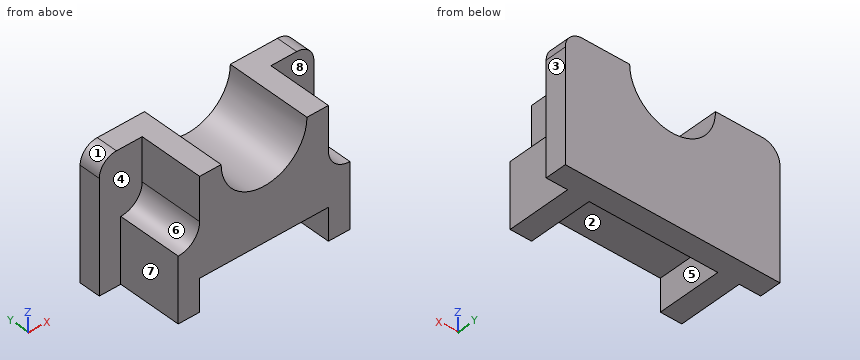
from build123d import *

# Parameters (mm, degrees)
F1_DEPTH = 6.35
F2_R     = 5.08
F4_DEPTH = 19.05
F5_DEPTH = 25.4
F6_DEPTH = 25.4
F7_DEPTH = 72.5614
F8_DEPTH = 61.46767


with BuildPart() as f1:
    # F0 (on Front) → F1 (new body)
    with BuildSketch(Plane.XZ):
        with BuildLine():
            Line((-25.4, 33.425663), (-44.45, 33.425663))
            Line((-44.45, 33.425663), (-44.45, -4.674337))
            Line((-44.45, -4.674337), (19.05, -4.674337))
            Line((19.05, -4.674337), (19.05, 33.425663))
            Line((19.05, 33.425663), (0, 33.425663))
            ThreePointArc((0, 33.425663), (-12.7, 20.725663), (-25.4, 33.425663))
        make_face()
        with BuildLine():
            Line((0, 33.425663), (-25.4, 33.425663))
            ThreePointArc((-25.4, 33.425663), (-12.7, 20.725663), (0, 33.425663))
        make_face()
    extrude(amount=F1_DEPTH)

    # F2
    f2_edges = [f1.edges().sort_by_distance(p)[0] for p in [
        (-44.45, -3.175, 33.425663),
        (19.05, -3.175, 33.425663),
    ]]
    fillet(f2_edges, radius=F2_R)

    # F3 (on face) → F4 (join)
    with BuildSketch(Plane.XZ.offset(6.35)):
        with BuildLine():
            Line((-38.1, 14.375663), (-38.1, -4.674337))
            Line((-38.1, -4.674337), (-31.75, -4.674337))
            Line((-31.75, -4.674337), (-31.75, 4.850663))
            Line((-31.75, 4.850663), (6.35, 4.850663))
            Line((6.35, 4.850663), (6.35, -4.674337))
            Line((6.35, -4.674337), (12.7, -4.674337))
            Line((12.7, -4.674337), (12.7, 14.375663))
            ThreePointArc((12.7, 14.375663), (8.209872, 16.235535), (6.35, 20.725663))
            Line((6.35, 20.725663), (6.35, 33.425663))
            Line((6.35, 33.425663), (-31.75, 33.425663))
            Line((-31.75, 33.425663), (-31.75, 20.725663))
            ThreePointArc((-31.75, 20.725663), (-33.609872, 16.235535), (-38.1, 14.375663))
        make_face()
        with BuildLine():
            Line((-38.1, 33.425663), (-38.1, 14.375663))
            ThreePointArc((-38.1, 14.375663), (-33.609872, 16.235535), (-31.75, 20.725663))
            Line((-31.75, 20.725663), (-31.75, 33.425663))
            Line((-31.75, 33.425663), (-38.1, 33.425663))
        make_face()
        with BuildLine():
            Line((12.7, 33.425663), (6.35, 33.425663))
            Line((6.35, 33.425663), (6.35, 20.725663))
            ThreePointArc((6.35, 20.725663), (8.209872, 16.235535), (12.7, 14.375663))
            Line((12.7, 14.375663), (12.7, 33.425663))
        make_face()
    extrude(amount=F4_DEPTH)

    # F0 (on Front) → F5 (cut)
    with BuildSketch(Plane.XZ):
        with BuildLine():
            Line((0, 33.425663), (-25.4, 33.425663))
            ThreePointArc((-25.4, 33.425663), (-12.7, 20.725663), (0, 33.425663))
        make_face()
    extrude(amount=-F5_DEPTH, mode=Mode.SUBTRACT)

    # F0 (on Front) → F6 (cut)
    with BuildSketch(Plane.XZ):
        with BuildLine():
            Line((0, 33.425663), (-25.4, 33.425663))
            ThreePointArc((-25.4, 33.425663), (-12.7, 20.725663), (0, 33.425663))
        make_face()
    extrude(amount=F6_DEPTH, mode=Mode.SUBTRACT)

    # F3 (on face) + F4_face (on face) → F7 (cut)
    with BuildSketch(Plane.XZ.offset(6.35)):
        with BuildLine():
            Line((-38.1, 33.425663), (-38.1, 14.375663))
            ThreePointArc((-38.1, 14.375663), (-33.609872, 16.235535), (-31.75, 20.725663))
            Line((-31.75, 20.725663), (-31.75, 33.425663))
            Line((-31.75, 33.425663), (-38.1, 33.425663))
        make_face()
    with BuildSketch(Plane(origin=(-12.7, -25.4, 15.682621), x_dir=(1, 0, 0), z_dir=(0, -1, 0))):
        with BuildLine():
            Line((-25.4, 17.743042), (-25.4, -20.356958))
            Line((-25.4, -20.356958), (-19.05, -20.356958))
            Line((-19.05, -20.356958), (-19.05, -10.831958))
            Line((-19.05, -10.831958), (19.05, -10.831958))
            Line((19.05, -10.831958), (19.05, -20.356958))
            Line((19.05, -20.356958), (25.4, -20.356958))
            Line((25.4, -20.356958), (25.4, 17.743042))
            Line((25.4, 17.743042), (12.7, 17.743042))
            ThreePointArc((12.7, 17.743042), (0, 5.043042), (-12.7, 17.743042))
            Line((-12.7, 17.743042), (-25.4, 17.743042))
        make_face()
    extrude(amount=F7_DEPTH, mode=Mode.SUBTRACT)

    # F3 (on face) → F8 (cut)
    with BuildSketch(Plane.XZ.offset(6.35)):
        with BuildLine():
            Line((12.7, 33.425663), (6.35, 33.425663))
            Line((6.35, 33.425663), (6.35, 20.725663))
            ThreePointArc((6.35, 20.725663), (8.209872, 16.235535), (12.7, 14.375663))
            Line((12.7, 14.375663), (12.7, 33.425663))
        make_face()
    extrude(amount=F8_DEPTH, mode=Mode.SUBTRACT)


solid = f1.part
For this review, take the finished solid that the model builds, in its own axes (mm). Face numbers are marked on the shaded views. A direction names the side the tool comes from. Give positions to 0.01 mm unless a question says otherwise; leave off trailing zeros. Loops run counter-clockwise (first coordinate to the right, second up) from the corner with the lowest first, then second, coordinate; pieces in that order, holes last. Notation, with made-up numbers: M -29.75,69 L 16.25,69 A15 cw 16.25,82 Z; hole C 68.25,35.5 d6. An arc over 180 degrees is marked long. Answer as a JSON object with one key per item and string values. Group by question number.
Q1. Mouldability with a two-part tool opening along X and no side actions: class the marked faces 1, 2, 3 and 4 as +X half, -X half, draft (parallel to the pull), parting line (faces both ways), or undercut.
Q2. Insertion check: P1, Ø10.5, axis at y = -13.5, z = -2, coming from the -X side; P2, Ø7.5, axis at y = -12.5, z = 2, coming from the +X side; P3, Ø4, axis at y = -18.5, z = 24.5, coming from the +X side. Each pin has a flat end and moves straight along its axis. Give the tip position at first contact, or say it passes through.
Q3. Add section A-A on z = 21.5. Give the boundary of the cut face in (x, y), and give its area (3 significant figures).
Q4. Add section C-C on x = -28.5. Give the boundary of the cut face in (y, z).
Q5. Add section B-B on y = -4. Give the boundary of the cut face in (x, z), and give its area (3 significant figures).
Q6. Tool access review of the marked faces 5, 6, 7 and 8: name each direction out of +Z, -Z, +X, -X, +Y, -Y from which nothing blocks a thin tool from reaching the whole face with its end or side.
Q7. Add section D-D on z = 2. Give the boundary of the cut face in (x, y), and give its area (3 significant figures).
Q8. For probe 1 along X at (y, z) = (-19, 3.5); probe 2 along Y at (x, z) = (-39.5, 27.5); probe 3 along Z at (x, y) = (-12.5, -8.5), list the stretches that pass through material, from the lowest coordinate up. Write a range as [from, to].
Checked values:
{
 "1": {"face 1": "-X half", "face 2": "undercut", "face 3": "+X half", "face 4": "draft"},
 "2": {"P1": "x = -38.1", "P2": "x = 12.7", "P3": "x = 6.35"},
 "3": {"outline": "M -44.45,-6.35 L -31.75,-6.35 L -31.75,-25.4 L -17.07,-25.4 L -17.07,0 L -44.45,0 Z; M -8.33,-25.4 L 6.35,-25.4 L 6.35,-6.35 L 19.05,-6.35 L 19.05,0 L -8.33,0 Z", "area": "907 mm²"},
 "4": {"outline": "M -25.4,4.85 L -6.35,4.85 L -6.35,-4.67 L 0,-4.67 L 0,33.43 L -25.4,33.43 Z"},
 "5": {"outline": "M -44.45,-4.67 L 19.05,-4.67 L 19.05,28.35 A5.08 ccw 13.97,33.43 L 0,33.43 A12.7 cw -25.4,33.43 L -39.37,33.43 A5.08 ccw -44.45,28.35 Z", "area": "2,150 mm²"},
 "6": {"face 5": "-Z, -Y", "face 6": "+Z, -X, -Y", "face 7": "+Z, -Z, -X, -Y", "face 8": "+Z, +X, -Y"},
 "7": {"outline": "M -44.45,-6.35 L -38.1,-6.35 L -38.1,-25.4 L -31.75,-25.4 L -31.75,-6.35 L 6.35,-6.35 L 6.35,-25.4 L 12.7,-25.4 L 12.7,-6.35 L 19.05,-6.35 L 19.05,0 L -44.45,0 Z", "area": "645 mm²"},
 "8": {"probe 1": "[-38.1, -31.75], [6.35, 12.7]", "probe 2": "[-6.35, 0]", "probe 3": "[4.85, 20.73]"}
}
